Autodesk Inventor part; units mm, degrees
ref_plane "YZ Plane" through (0, 0, 0) normal (1, 0, 0) x (0, 1, 0)
ref_plane "XZ Plane" through (0, 0, 0) normal (0, 1, 0) x (-1, 0, 0)
ref_plane "XY Plane" through (0, 0, 0) normal (0, 0, 1) x (1, 0, 0)
sketch "Sketch1" plane through (0, 0, 0) normal (0, 0, 1) x (1, 0, 0)
  line L0 (0, 46) -> (0, 0)
  line L1 (0, 0) -> (28, 0)
  line L2 (28, 0) -> (28, 10)
  line L3 (0, 46) -> (10, 46)
  line L4 (10, 46) -> (28, 10)
  dimension "d0" = 10
  dimension "d1" = 10
  dimension "d2" = 46
  dimension "d3" = 28
extrude "Extrusion1" add sketch "Sketch1" along normal blind 6
sketch "Sketch2" plane through (0, 0, 6) normal (0, 0, 1) x (1, 0, 0)
  line L0 (0, 46) -> (0, 0)
  line L1 (0, 0) -> (28, 0)
  line L2 (0, 43) -> (-4, 43)
  line L3 (-6, 41) -> (-6, 37)
  line L4 (-4, 35) -> (0, 35)
  line L5 (0, 35) -> (0, 43)
  line L6 (0, 20) -> (-4, 20)
  line L7 (-6, 18) -> (-6, 14)
  line L8 (-4, 12) -> (0, 12)
  line L9 (0, 12) -> (0, 20)
  line L10 (16, 0) -> (24, 0)
  line L11 (24, 0) -> (24, -4)
  line L12 (22, -6) -> (18, -6)
  line L13 (16, -4) -> (16, 0)
  arc A0 (-4, 43) -> (-6, 41) centre (-4, 41) ccw
  arc A1 (-6, 37) -> (-4, 35) centre (-4, 37) ccw
  arc A2 (-4, 20) -> (-6, 18) centre (-4, 18) ccw
  arc A3 (-6, 14) -> (-4, 12) centre (-4, 14) ccw
  arc A4 (16, -4) -> (18, -6) centre (18, -4) ccw
  arc A5 (22, -6) -> (24, -4) centre (22, -4) ccw
  line L14 (28, 0) -> (28, 10)
  point P0 (-6, 35)
  point P1 (-6, 43)
  point P2 (-6, 12)
  point P3 (-6, 20)
  point P4 (24, -6)
  point P5 (16, -6)
  dimension "d6" = 8
  dimension "d7" = 8
  dimension "d9" = 8
  dimension "d10" = 12
  dimension "d11" = 15
  dimension "d15" = 2
  dimension "d16" = 6
  dimension "d38" = 4
  dimension "d39" = 6
sketch "Sketch3" plane through (0, 0, 6) normal (0, 0, 1) x (1, 0, 0)
  line L0 (0, 0) -> (28, 0)
  line L1 (6.5, 0) -> (6.5, 5)
  line L2 (6.5, 5) -> (4, 5)
  line L3 (4, 5) -> (4, 12.3)
  line L4 (4, 12.3) -> (6.5, 12.3)
  line L5 (6.5, 12.3) -> (6.5, 16.3)
  line L6 (6.5, 16.3) -> (11, 16.3)
  line L7 (11, 16.3) -> (11, 12.3)
  line L8 (11, 12.3) -> (13.5, 12.3)
  line L9 (13.5, 12.3) -> (13.5, 5)
  line L10 (13.5, 5) -> (11, 5)
  line L11 (11, 5) -> (11, 0)
  line L12 (0, 46) -> (0, 0)
  point P0 (11, 0)
  point P1 (26, 0)
  point P2 (8.75, 16.3)
  dimension "d27" = 4.5
  dimension "d28" = 5
  dimension "d29" = 7.3
  dimension "d30" = 4
  dimension "d32" = 2.5
  dimension "d33" = 2.5
  dimension "d41" = 4
extrude "Extrusion4" cut sketch "Sketch3" against normal through all
extrude "Extrusion5" add sketch "Sketch2" against normal blind 6
properties part number "x_carryage_brace"
Design review of the part built by this model. Coordinates are the model's own, in mm. A direction names the side the tool comes from. Coordinates: 2 decimals unless noted, no trailing zeros. Loops run counter-clockwise (first coordinate to the right, second up) from the corner with the lowest first, then second, coordinate; pieces in that order, holes last. Notation, with made-up numbers: M 74.25,-39 L 108.25,-39 A13 cw 108.25,-33 Z; hole C 27,-14.5 d10. An arc over 180 degrees is marked long. One line per question, with ' | ' between items.
(1) Machinability: for faces 1 (the face through (6.5, 14, 3)), 2 (the face through (-2, 43, 3)), 3 (the face through (12, 12.3, 3)), 4 (the face through (16, -2, 3)), which of the approach directions +Z, -Z, +X, -X, +Y, -Y give a long, thin tool a straight path to every point of the face, cutting with its end or side? Answer none if there is none.
Filled in:
face 1: +Z, -Z, -Y | face 2: +Z, -Z, -X, +Y | face 3: +Z, -Z | face 4: +Z, -Z, -X, -Y
(2) We need section A-A (y = 14.5). Give the boundary of the cut face in (x, z), and give its area (4 significant figures).
Filled in:
outline: M -6,0 L 6.5,0 L 6.5,6 L -6,6 Z; M 11,0 L 25.75,0 L 25.75,6 L 11,6 Z | area: 163.5 mm^2
(3) Draft analysis for pull direction Y (two halves, no side actions). For faces 5 (the face through (0, 6, 3)), 6 (the face through (5, 5, 3)), 7 (the face through (19, 28, 3)), state which applies: released by +Y, released by -Y, zero draft, split by the parting line, or undercut.
Filled in:
face 5: zero draft | face 6: undercut | face 7: released by +Y
(4) Wall thickness on probe 1 along Y at (x, z) = (-1, 4); probe 2 along Y at (x, z) = (5.5, 4.85); probe 3 along X at (y, z) = (8.5, 3.8): over which ranges is each line inside the solid? List them lowest first.
Filled in:
probe 1: y = 12 to 20, 35 to 43 | probe 2: y = 0 to 5, 12.3 to 46 | probe 3: x = 0 to 4, 13.5 to 28
(5) For pin 1 Ø2 at (x, z) = (26, 2.5) entering from -Y; pin 2 Ø3 at (y, z) = (14, 4) entering from +X; pin 3 Ø2 at (y, z) = (24.5, 4) entering from +X, all flat-tipped, find the tip position at first contact; note any pin that passes through.
Filled in:
pin 1: stops at y = 0 | pin 2: stops at x = 26.75 | pin 3: stops at x = 21.25
(6) We need section C-C (x = 8). Give the boundary of the cut face in (y, z).
Filled in:
outline: M 16.3,0 L 46,0 L 46,6 L 16.3,6 Z
(7) We need section D-D (y = 29). Give the boundary of the cut face in (x, z), and give its area (3 significant figures).
Filled in:
outline: M 0,0 L 18.5,0 L 18.5,6 L 0,6 Z | area: 111 mm^2
(8) We need section B-B (y = 4). Give the boundary of the cut face in (x, z).
Filled in:
outline: M 0,0 L 6.5,0 L 6.5,6 L 0,6 Z; M 11,0 L 28,0 L 28,6 L 11,6 Z
